Verification items for the finished model (mm, model axes). A direction names the side the tool comes from. Coordinates: 2 decimals unless noted, no trailing zeros. Order: outer loops, then holes, each group sorted by start corner. A loop starts at its lowest first (then second) coordinate and runs counter-clockwise, first axis right, second up. Notation, with made-up numbers: M 68,62 L 108,62 A21 cw 108,72 Z; hole C -40,77.5 d10. An arc over 180 degrees is marked long. Write item = value, one per line.
Autodesk Inventor part; units mm, degrees
ref_plane "YZ Plane" through (0, 0, 0) normal (1, 0, 0) x (0, 1, 0)
ref_plane "XZ Plane" through (0, 0, 0) normal (0, 1, 0) x (-1, 0, 0)
ref_plane "XY Plane" through (0, 0, 0) normal (0, 0, 1) x (1, 0, 0)
sketch "스케치1" plane through (0, 0, 0) normal (1, 0, 0) x (0, 1, 0)
  circle A0 centre (0, 0) radius 1.65
  line L0 (-23.6101, -11.5918) -> (-23.6101, -7.0918)
  arc A1 (3.6862, -2.5811) -> (-3.6862, 2.5811) centre (0, 0) ccw
  line L1 (-3.6862, 2.5811) -> (-10.4592, -7.0918)
  line L2 (-10.4592, -7.0918) -> (-23.6101, -7.0918)
  line L3 (3.6862, -2.5811) -> (-2.6232, -11.5918)
  line L4 (-2.6232, -11.5918) -> (-23.6101, -11.5918)
  line L5 (-10.4592, -7.0918) -> (-9.0498, -7.0918)
  line L6 (-9.0498, -7.0918) -> (-9.0498, -11.5918)
  dimension "d5" = 4.5
extrude "돌출1" add sketch "스케치1" along normal blind 36 contours A0 | L0 L2 L5 L6 L4 | L6 L5 L1 A1 L3 L4
sketch "스케치4" plane through (0, -23.6101, -11.5918) normal (0, 0, -1) x (-1, 0, 0)
  line L0 (-36, 14.5515) -> (-31, 14.5515)
  line L1 (-31, 14.5515) -> (-30, 14.5515)
  line L2 (-30, 14.5515) -> (-21.5, 14.5515)
  line L3 (-21.5, 14.5515) -> (-20.5, 14.5515)
  line L4 (-20.5, 14.5515) -> (-15.5, 14.5515)
  line L5 (-15.5, 14.5515) -> (-14.5, 14.5515)
  line L6 (-14.5, 14.5515) -> (-6, 14.5515)
  line L7 (-6, 14.5515) -> (-5, 14.5515)
  line L8 (-5, 14.5515) -> (0, 14.5515)
  line L9 (-36, 14.5515) -> (-36, 28.1225)
  line L10 (-36, 28.1225) -> (-31, 28.1225)
  line L11 (-31, 28.1225) -> (-31, 14.5515)
  line L12 (-31, 14.5515) -> (-36, 14.5515)
  line L13 (-36, 19.9239) -> (-36, 13.1509)
  line L14 (-31, 28.1225) -> (-30, 28.1225)
  line L15 (-30, 28.1225) -> (-30, 14.5515)
  line L16 (-30, 14.5515) -> (-31, 14.5515)
  line L17 (-31, 14.5515) -> (-31, 28.1225)
  line L18 (-30, 28.1225) -> (-21.5, 28.1225)
  line L19 (-21.5, 28.1225) -> (-21.5, 14.5515)
  line L20 (-21.5, 14.5515) -> (-30, 14.5515)
  line L21 (-30, 14.5515) -> (-30, 28.1225)
  line L22 (-21.5, 28.1225) -> (-20.5, 28.1225)
  line L23 (-20.5, 28.1225) -> (-20.5, 14.5515)
  line L24 (-20.5, 14.5515) -> (-21.5, 14.5515)
  line L25 (-21.5, 14.5515) -> (-21.5, 28.1225)
  line L26 (-20.5, 28.1225) -> (-15.5, 28.1225)
  line L27 (-15.5, 28.1225) -> (-15.5, 14.5515)
  line L28 (-15.5, 14.5515) -> (-20.5, 14.5515)
  line L29 (-20.5, 14.5515) -> (-20.5, 28.1225)
  line L30 (-15.5, 28.1225) -> (-14.5, 28.1225)
  line L31 (-14.5, 28.1225) -> (-14.5, 14.5515)
  line L32 (-14.5, 14.5515) -> (-15.5, 14.5515)
  line L33 (-15.5, 14.5515) -> (-15.5, 28.1225)
  line L34 (-14.5, 28.1225) -> (-6, 28.1225)
  line L35 (-6, 28.1225) -> (-6, 14.5515)
  line L36 (-6, 14.5515) -> (-14.5, 14.5515)
  line L37 (-14.5, 14.5515) -> (-14.5, 28.1225)
  line L38 (-6, 28.1225) -> (-5, 28.1225)
  line L39 (-5, 28.1225) -> (-5, 14.5515)
  line L40 (-5, 14.5515) -> (-6, 14.5515)
  line L41 (-6, 14.5515) -> (-6, 28.1225)
  line L42 (-5, 28.1225) -> (0, 28.1225)
  line L43 (0, 28.1225) -> (0, 14.5515)
  line L44 (0, 14.5515) -> (-5, 14.5515)
  line L45 (-5, 14.5515) -> (-5, 28.1225)
  line L46 (-36, 13.1509) -> (-10.5, 13.1509)
  line L47 (0, 13.1509) -> (-36, 13.1509)
  line L48 (-18, 13.1509) -> (-18, 6.1509)
  line L49 (-18, 6.1509) -> (-25.5, 6.1509)
  line L50 (-18, 6.1509) -> (-10.5, 6.1509)
  circle A0 centre (-25.5, 6.1509) radius 2.65
  circle A1 centre (-10.5, 6.1509) radius 2.65
  dimension "d17" = 5
  dimension "d18" = 1
  dimension "d19" = 8.5
  dimension "d20" = 1
  dimension "d21" = 5
  dimension "d22" = 1
  dimension "d23" = 8.5
  dimension "d24" = 1
  dimension "d25" = 5
  dimension "d38" = 7
  dimension "d39" = 7.5
  dimension "d40" = 7.5
  dimension "d41" = 5.3
  dimension "d42" = 5.3
extrude "돌출2" cut sketch "스케치4" against normal blind 18 contours L11 L14 L15 L1 | L15 L18 L19 L2 | L19 L22 L23 L3 | L27 L30 L31 L5 | L31 L34 L35 L6 | L35 L38 L39 L7
extrude "돌출3" cut sketch "스케치1" along normal blind 36 contours A0
extrude "돌출6" cut sketch "스케치4" against normal blind 10 contours A0
extrude "돌출7" cut sketch "스케치4" against normal blind 10 contours A1
properties part number "xy 아이들러"
Item 1: Sectioned sample at B-B, the plane z = -4.5. Enter the section's corners in (x, y), then the cut area to 3 significant figures.
Report:
outline = M 0,-8.64 L 5,-8.64 L 5,2.34 L 0,2.34 Z; M 15.5,-8.64 L 20.5,-8.64 L 20.5,2.34 L 15.5,2.34 Z; M 31,-8.64 L 36,-8.64 L 36,2.34 L 31,2.34 Z
area = 165 mm^2
Item 2: Sectioned sample at D-D, the plane z = -9.75. Enter the section's corners in (x, y), then the cut area to 3 significant figures.
Report:
outline = M 0,-23.61 L 36,-23.61 L 36,-1.33 L 31,-1.33 L 31,-9.06 L 20.5,-9.06 L 20.5,-1.33 L 15.5,-1.33 L 15.5,-9.06 L 5,-9.06 L 5,-1.33 L 0,-1.33 Z; hole C 10.5,-17.46 d5.3; hole C 25.5,-17.46 d5.3
area = 596 mm^2
Item 3: Tool access check on faces 4 (the flat face through (18, -17, -7.092)), 5 (the flat face through (15.5, -2, -4)), 6 (the cylindrical face through (25.84, -14.83, -9.37)). Record the directions out of +Z, -Z, +X, -X, +Y, -Y that give a thin tool (end or side, any length) a straight path to the whole face; none if there is none.
Report:
face_4 = +Z, +X, -X, -Y
face_5 = +Z, -Z, +Y
face_6 = +Z, -Z
Item 4: Release check for a two-part mould opening along X. For faces 1 (the flat face through (0, -7, -5)), 2 (the flat face through (18, -23.61, -9)), 3 (the flat face through (10, -9.059, -8)) record: pulls with the +X half, pulls with the -X half, needs draft (parallel to the pull), parting line crosses it, or undercut.
Report:
face_1 = pulls with the -X half
face_2 = needs draft
face_3 = undercut
Item 5: Sectioned sample at A-A, the plane x = 25.5. Enter the section's corners in (y, z).
Report:
outline = M -23.61,-11.59 L -20.11,-11.59 L -20.11,-7.09 L -23.61,-7.09 Z; M -14.81,-11.59 L -9.06,-11.59 L -9.06,-5.09 L -10.46,-7.09 L -14.81,-7.09 Z
Item 6: Sectioned sample at C-C, the plane y = 0. Enter the section's corners in (x, z), then the cut area to 3 significant figures.
Report:
outline = M 0,-7.85 L 5,-7.85 L 5,-1.65 L 0,-1.65 Z; M 0,1.65 L 5,1.65 L 5,4.5 L 0,4.5 Z; M 15.5,-7.85 L 20.5,-7.85 L 20.5,-1.65 L 15.5,-1.65 Z; M 15.5,1.65 L 20.5,1.65 L 20.5,4.5 L 15.5,4.5 Z; M 31,-7.85 L 36,-7.85 L 36,-1.65 L 31,-1.65 Z; M 31,1.65 L 36,1.65 L 36,4.5 L 31,4.5 Z
area = 136 mm^2
Item 7: Scan lines: L1, parallel to X at y = -4, z = -8.75; L2, parallel to X at y = -17.5, z = -10; L3, parallel to Y at x = 10.5, z = -8.3. Record each from-to range of solid material in increasing order. Write a range as from..to.
Report:
L1 = 0..5, 15.5..20.5, 31..36
L2 = 0..7.85, 13.15..22.85, 28.15..36
L3 = -23.61..-20.11, -14.81..-9.06
Item 8: Gauge pin test, flat ends, axial feed: pin 1 (1 mm diameter, centred on x = 10, y = -12.5, fed in from +Z); pin 2 (3 mm diameter, centred on x = 13.5, y = 0, fed in from -Z); pin 3 (2 mm diameter, centred on x = 10.5, z = -8.5, fed in from +Y); pin 4 (4 mm diameter, centred on x = 20, y = 1, fed in from -Z). Record the tip position at first contact, or that the pin passes through.
Report:
pin_1 = -7.09
pin_2 = through
pin_3 = -9.06
pin_4 = -9.27
